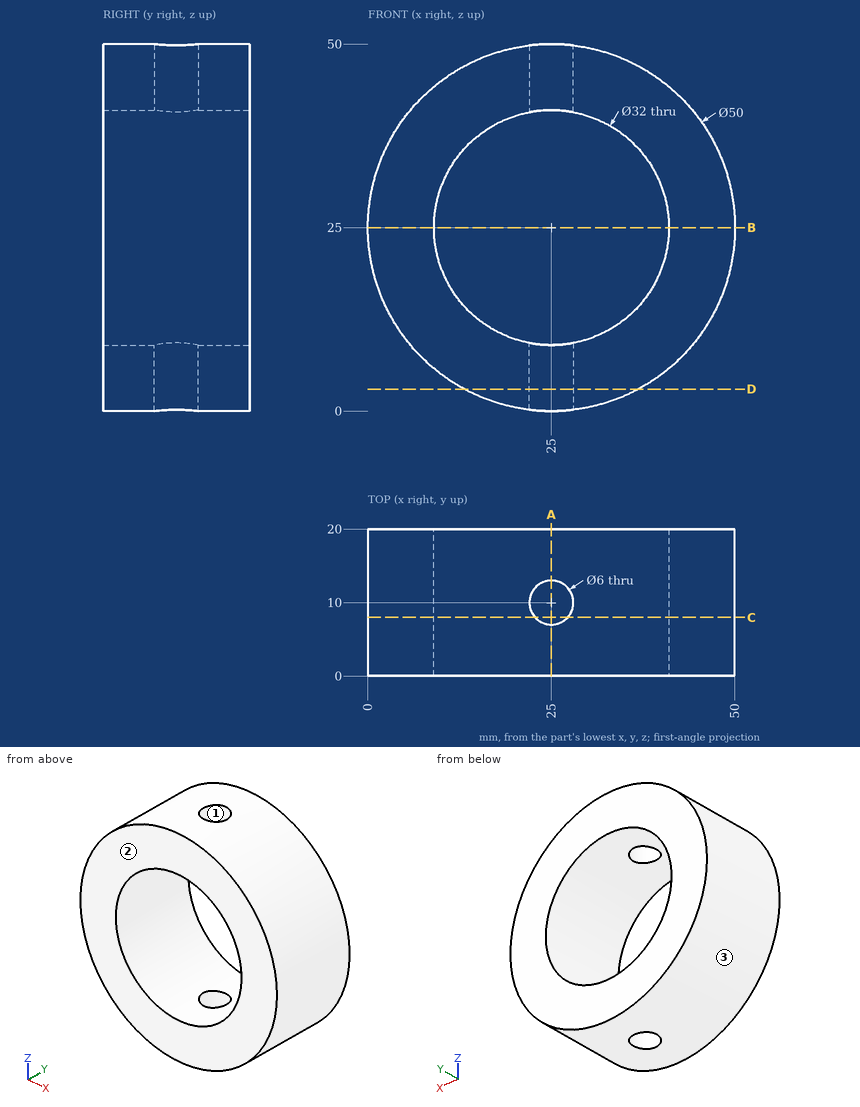
The figure shows three views and two pictorial views of one solid part (mm, origin at its lowest corner). Answer the questions. Coordinates: 2 decimals unless noted, no trailing zeros. Write each loop counter-clockwise with the first axis right and the second up, starting at its lowest first coordinate (ties: lowest second). Pieces come first, ordered by that corner, then holes.
1. Flat-ended cylindrical pins translate along their axes: pin 1 (2 mm diameter, centred on y = 14.5, z = 38.5, fed in from -X); pin 2 (5.5 mm diameter, centred on x = 25, y = 10, fed in from +Z); pin 3 (3 mm diameter, centred on x = 22.5, y = 5, fed in from -Z); pin 4 (8 mm diameter, centred on x = 31, y = 9, fed in from -Z). Find the tip coordinate at first contact, or state that the pin passes through.
Results list:
pin 1: stops at x = 3.35
pin 2: passes through
pin 3: stops at z = 0.02
pin 4: stops at z = 0.09
2. Consider line 1 along Y through (x, z) = (25, 3); line 2 along X through (y, z) = (2, 32); line 3 along Z through (x, y) = (29, 11.5). Determine where each line is inside the solid, lowest interval first.
Results list:
line 1: y = 0 to 7, 13 to 20
line 2: x = 1 to 10.61, 39.39 to 49
line 3: z = 0.32 to 9.51, 40.49 to 49.68
3. For a pull along X with two mould halves and no side action, classify the marked faces 1, 2 and 3 as +X half, -X half, draft (parallel to the pull), parting line (faces both ways), or undercut.
Results list:
face 1: undercut
face 2: draft
face 3: parting line
4. The part is cut by section C-C, the plane y = 8. Write down the section's boundary in (x, z), and give its area (3 significant figures).
Results list:
outline: (22.76, 0.1) - (22.76, 9.16) arc R16 cw to (22.76, 40.84) - (22.76, 49.9) arc R25 ccw to start; (27.24, 0.1) arc R25 ccw to (27.24, 49.9) - (27.24, 40.84) arc R16 cw to (27.24, 9.16) - close
area: 1,080 mm2
5. The part is cut by section D-D, the plane z = 3. Write down the section's boundary in (x, y).
Results list:
outline: (13.13, 0) - (36.87, 0) - (36.87, 20) - (13.13, 20) - close; hole circle Ø6 at (25, 10)
6. The part is cut by section B-B, the plane z = 25. Write down the section's boundary in (x, y).
Results list:
outline: (0, 0) - (9, 0) - (9, 20) - (0, 20) - close; (41, 0) - (50, 0) - (50, 20) - (41, 20) - close
7. The part is cut by section A-A, the plane x = 25. Write down the section's boundary in (y, z), and give its area (3 significant figures).
Results list:
outline: (0, 0) - (7, 0) - (7, 9) - (0, 9) - close; (0, 41) - (7, 41) - (7, 50) - (0, 50) - close; (13, 0) - (20, 0) - (20, 9) - (13, 9) - close; (13, 41) - (20, 41) - (20, 50) - (13, 50) - close
area: 252 mm2
